```python
from build123d import *

# Parameters (mm, degrees)
SERVO_SHELF_START                 = 21.4
SERVO_SHELF_PROFILE_W             = 46
SERVO_SHELF_PROFILE_H             = 36
SERVO_SHELF_DEPTH                 = 4
REAR_CLAMPING_BLOCK_START         = -18
REAR_CLAMPING_BLOCK_PROFILE_W     = 7
REAR_CLAMPING_BLOCK_PROFILE_H     = 10
REAR_CLAMPING_BLOCK_DEPTH         = 36
SERVO_BODY_WINDOW_START           = 20.4
SERVO_BODY_WINDOW_PROFILE_W       = 23.8
SERVO_BODY_WINDOW_PROFILE_H       = 13
SERVO_BODY_WINDOW_DEPTH           = 25.744213361
LEFT_NUT_ACCESS_START             = 20
LEFT_NUT_ACCESS_PROFILE_W         = 10
LEFT_NUT_ACCESS_PROFILE_H         = 8
LEFT_NUT_ACCESS_DEPTH             = 26.144213361
RIGHT_NUT_ACCESS_START            = 20
RIGHT_NUT_ACCESS_PROFILE_W        = 10
RIGHT_NUT_ACCESS_PROFILE_H        = 8
RIGHT_NUT_ACCESS_DEPTH            = 26.144213361
REAR_CLAMPING_M3_HOLES_START      = -25
REAR_CLAMPING_M3_PROFILE_R        = 1.6
REAR_CLAMPING_M3_HOLES_DEPTH      = 11
FILLET1_R                         = 3
FILLET2_R                         = 1
BOSS_EXTRUDE1_START               = -36
BOSS_EXTRUDE1_DEPTH               = 36
OWNED_SG90_M2_EAR_HOLES_START     = 20.4
OWNED_SG90_M2_EAR_HOLES_PROFILE_R = 1.2
OWNED_SG90_M2_EAR_HOLES_DEPTH     = 25.744213361


with BuildPart() as part:
    # Servo_shelf_profile → Servo_shelf (new body)
    with BuildSketch(Plane(origin=(0, 0, 0), x_dir=(1, 0, 0), z_dir=(0, 1, 0)).offset(SERVO_SHELF_START)):
        with Locations((2, 0)):
            Rectangle(SERVO_SHELF_PROFILE_W, SERVO_SHELF_PROFILE_H)
    extrude(amount=SERVO_SHELF_DEPTH)

    # Rear_clamping_block_profile → Rear_clamping_block (add)
    with BuildSketch(Plane.XY.offset(REAR_CLAMPING_BLOCK_START)):
        with Locations((-17.5, 28)):
            Rectangle(REAR_CLAMPING_BLOCK_PROFILE_W, REAR_CLAMPING_BLOCK_PROFILE_H)
    extrude(amount=REAR_CLAMPING_BLOCK_DEPTH)

    # Servo_body_window_profile → Servo_body_window (cut, through all)
    with BuildSketch(Plane(origin=(0, 0, 0), x_dir=(1, 0, 0), z_dir=(0, 1, 0)).offset(SERVO_BODY_WINDOW_START)):
        with Locations((5.5, 0)):
            Rectangle(SERVO_BODY_WINDOW_PROFILE_W, SERVO_BODY_WINDOW_PROFILE_H)
    extrude(amount=SERVO_BODY_WINDOW_DEPTH, mode=Mode.SUBTRACT)

    # Left_nut_access_profile → Left_nut_access (cut, through all)
    with BuildSketch(Plane(origin=(0, 0, 0), x_dir=(1, 0, 0), z_dir=(0, 1, 0)).offset(LEFT_NUT_ACCESS_START)):
        with Locations((-9, 12)):
            Rectangle(LEFT_NUT_ACCESS_PROFILE_W, LEFT_NUT_ACCESS_PROFILE_H)
    extrude(amount=LEFT_NUT_ACCESS_DEPTH, mode=Mode.SUBTRACT)

    # Right_nut_access_profile → Right_nut_access (cut, through all)
    with BuildSketch(Plane(origin=(0, 0, 0), x_dir=(1, 0, 0), z_dir=(0, 1, 0)).offset(RIGHT_NUT_ACCESS_START)):
        with Locations((-9, -12)):
            Rectangle(RIGHT_NUT_ACCESS_PROFILE_W, RIGHT_NUT_ACCESS_PROFILE_H)
    extrude(amount=RIGHT_NUT_ACCESS_DEPTH, mode=Mode.SUBTRACT)

    # Rear_clamping_M3_profile → Rear_clamping_M3_holes (cut)
    with BuildSketch(Plane(origin=(0, 0, 0), x_dir=(0, 0, -1), z_dir=(1, 0, 0)).offset(REAR_CLAMPING_M3_HOLES_START)):
        with Locations((12, 28)):
            Circle(REAR_CLAMPING_M3_PROFILE_R)
        with Locations((-12, 28)):
            Circle(REAR_CLAMPING_M3_PROFILE_R)
    extrude(amount=REAR_CLAMPING_M3_HOLES_DEPTH, mode=Mode.SUBTRACT)

    # Fillet1
    fillet1_edges = [part.edges().sort_by_distance(p)[0] for p in [
        (-4, 23.4, -8),
        (-4, 23.4, -16),
        (-4, 23.4, 16),
        (-4, 23.4, 8),
    ]]
    fillet(fillet1_edges, radius=FILLET1_R)

    # Fillet2
    fillet2_edges = [part.edges().sort_by_distance(p)[0] for p in [
        (5.5, 25.4, 18),
        (-14, 25.4, 17),
        (5.5, 25.4, -18),
        (-14, 29.2, 18),
        (-14, 29.2, -18),
        (-14, 25.4, -17),
        (-14, 23.4, -16),
        (-14, 23.4, 16),
    ]]
    fillet(fillet2_edges, radius=FILLET2_R)

    # Sketch1 → Boss-Extrude1 (add)
    with BuildSketch(Plane(origin=(0, 0, -18), x_dir=(-1, 0, 0), z_dir=(0, 0, -1)).offset(BOSS_EXTRUDE1_START)):
        Polygon((14, 21.4), (21, 15), (21, 21.4), align=None)
    extrude(amount=BOSS_EXTRUDE1_DEPTH)

    # Owned_SG90_M2_ear_holes_profile → Owned_SG90_M2_ear_holes (cut, through all)
    with BuildSketch(Plane(origin=(0, 0, 0), x_dir=(1, 0, 0), z_dir=(0, 1, 0)).offset(OWNED_SG90_M2_EAR_HOLES_START)):
        with Locations(Location((-8.4, 0, 0), (0, 0, 90))):
            Circle(OWNED_SG90_M2_EAR_HOLES_PROFILE_R)
        with Locations(Location((19.4, 0, 0), (0, 0, 90))):
            Circle(OWNED_SG90_M2_EAR_HOLES_PROFILE_R)
    extrude(amount=OWNED_SG90_M2_EAR_HOLES_DEPTH, mode=Mode.SUBTRACT)


solid = part.part
```
The model under review builds one solid part; all positions refer to its coordinate system, in mm. A direction names the side the tool comes from. Give positions to 0.01 mm unless a question says otherwise; leave off trailing zeros. Write each loop counter-clockwise with the first axis right and the second up, starting at its lowest first coordinate (ties: lowest second). Pieces come first, ordered by that corner, then holes. Notation, with made-up numbers: M 17,18 L 21,18 A15 cw 21,35 Z; hole C 18,-18 d4. An arc over 180 degrees is marked long. Write item = value, one per line. Start each with the question number.
Q1. Mouldability with a two-part tool opening along Z and no side actions: class faces 6 (the face through (25, 23, 0)), 7 (the face through (-10, 23, 16)), 8 (the face through (-5, 23, 18)) as released by +Z, released by -Z, zero draft, split by the parting line, or undercut.
Q2. We need section D-D (x = -8.4). State the section outline as (y, z) points, plus the area to 3 significant figures.
Q3. We need section C-C (z = 0). State the section outline as (x, y) points.
Q4. We need section A-A (z = 12). State the section outline as (x, y) points, plus the area to 3 significant figures.
Q5. For line 1 (Z direction, x = -18, y = 28); line 2 (X direction, y = 24.65, z = 0); line 3 (Z direction, x = 5, y = 24.5), list the stretches that pass through material, from the lowest coordinate up.
Q6. We need section B-B (x = 19.4). State the section outline as (y, z) points.
Q7. Clearance check with flat-ended pins moving along their axes: pin 1 (2 mm diameter, centred on x = -8.4, z = 0, fed in from -Y); pin 2 (8 mm diameter, centred on x = -5, y = 24.5, fed in from -Z); pin 3 (10 mm diameter, centred on x = 15, z = 2.5, fed in from -Y); pin 4 (8 mm diameter, centred on x = 19, y = 29, fed in from -Z). State where each tip first meets the part, or that it passes through.
Q8. Machinability: for faces 1 (the face through (5, 21.4, -8)), 2 (the face through (6.266, 25.099, 17.715)), 3 (the face through (-14, 28, 0)), 4 (the face through (-21, 24, 0)), 5 (the face through (-11, 23, -8)), which of the approach directions +Z, -Z, +X, -X, +Y, -Y give a long, thin tool a straight path to every point of the face, cutting with its end or side? Answer none if there is none.
Result set:
q1.face_6 = zero draft
q1.face_7 = undercut
q1.face_8 = released by +Z
q2.outline = M 21.4,-18 L 24.4,-18 A1 ccw 25.4,-17 L 25.4,-16 L 21.4,-16 Z; M 21.4,-8 L 25.4,-8 L 25.4,-1.2 L 21.4,-1.2 Z; M 21.4,1.2 L 25.4,1.2 L 25.4,8 L 21.4,8 Z; M 21.4,16 L 25.4,16 L 25.4,17 A1 ccw 24.4,18 L 21.4,18 Z
q2.area = 70.0 mm2
q3.outline = M -21,15 L -14,21.4 L -9.6,21.4 L -9.6,25.4 L -14,25.4 L -14,33 L -21,33 Z; M -7.2,21.4 L -6.4,21.4 L -6.4,25.4 L -7.2,25.4 Z; M 17.4,21.4 L 18.2,21.4 L 18.2,25.4 L 17.4,25.4 Z; M 20.6,21.4 L 25,21.4 L 25,25.4 L 20.6,25.4 Z
q4.outline = M -21,15 L -14,21.4 L -14,26.4 L -21,26.4 Z; M -21,29.6 L -14,29.6 L -14,33 L -21,33 Z; M -4,21.4 L 25,21.4 L 25,25.4 L -4,25.4 Z
q4.area = 197 mm2
q5.line_1 = -18 to -13.6, -10.4 to 10.4, 13.6 to 18
q5.line_2 = -21 to -9.6, -7.2 to -6.4, 17.4 to 18.2, 20.6 to 25
q5.line_3 = -17.99 to -6.5, 6.5 to 17.99
q6.outline = M 21.4,-18 L 24.4,-18 A1 ccw 25.4,-17 L 25.4,-1.2 L 21.4,-1.2 Z; M 21.4,1.2 L 25.4,1.2 L 25.4,17 A1 ccw 24.4,18 L 21.4,18 Z
q7.pin_1 = through
q7.pin_2 = -18
q7.pin_3 = 21.4
q7.pin_4 = -17.8
q8.face_1 = +Z, -Z, +X, -Y
q8.face_2 = +Z, +X, +Y
q8.face_3 = +Y
q8.face_4 = +Z, -Z, -X, +Y, -Y
q8.face_5 = +Y, -Y
